```python
from build123d import *

# Parameters (mm, degrees)
F2_DEPTH = 12.7
F3_R     = 1.5875
F4_DEPTH = 12.701


# Not quite as in the source:
# - a feature names something its author has since deleted; it is built from what else it names


with BuildPart() as f2:
    # F1 (on face) → F2 (new body)
    with BuildSketch(Plane.YZ):
        Polygon((-152.4, -76.2), (139.7, -76.2), (139.7, 0), (152.4, 0), (152.4, 76.2), (-152.4, 76.2), (-207.8690637022, 76.2), align=None)
    extrude(amount=F2_DEPTH)

    # F3 (on face) → F4 (cut, through all)
    with BuildSketch(Plane.YZ):
        with Locations((-141.2875, 0)):
            Circle(F3_R)
        with Locations((88.9, 0)):
            Circle(F3_R)
    extrude(amount=F4_DEPTH, mode=Mode.SUBTRACT)


solid = f2.part
```
Could you check a few things on this model? Use its own coordinates, in mm. A direction names the side the tool comes from. Coordinates: 2 decimals unless noted, no trailing zeros. Write each loop counter-clockwise with the first axis right and the second up, starting at its lowest first coordinate (ties: lowest second). Pieces come first, ordered by that corner, then holes. Notation, with made-up numbers: (68, 49) - (110, 49) arc R23 ccw to (110, 67) - close; hole circle Ø10 at (75, 77). An arc over 180 degrees is marked (long way). Use a Markdown table: item, result.
Q1. Imagine slicing it at B-B (z = 41). List the corners of the cut face in (x, y) for me, and give its area (3 significant figures).
Geometry check:
| item | result |
|---|---|
| outline | (0, -195.06) - (12.7, -195.06) - (12.7, 152.4) - (0, 152.4) - close |
| area | 4,410 mm2 |
Q2. Which directions (+Z, -Z, +X, -X, +Y, -Y) give clear straight access to the entire face, cutting with the end or side of a thin tool? Please do faces 1 (the flat face through (0, -30, 1)), 2 (the flat face through (6, 139.7, -39)).
Geometry check:
| item | result |
|---|---|
| face 1 | +Z, -Z, -X, +Y, -Y |
| face 2 | -Z, +X, -X, +Y |
Q3. I'm going to push flat-ended pins straight in: pin 1 Ø3.5 at (y, z) = (88.9, 0) entering from -X; pin 2 Ø3 at (x, z) = (7.5, -4) entering from -Y; pin 3 Ø4 at (x, z) = (4.5, -47.5) entering from +Y; pin 4 Ø3 at (x, z) = (2.5, -57.5) entering from -Y. Where does each tip first touch, or does it pass through?
Geometry check:
| item | result |
|---|---|
| pin 1 | stops at x = 0 |
| pin 2 | stops at y = -179.22 |
| pin 3 | stops at y = 139.7 |
| pin 4 | stops at y = -159.75 |
Q4. Please list where these lines run through material, in increasing order: L1, parallel to Z at x = 10, y = 88.9; L2, parallel to Y at x = 7.25, z = 18; L3, parallel to Y at x = 7.5, z = 44.
Geometry check:
| item | result |
|---|---|
| L1 | z = -76.2 to -1.59, 1.59 to 76.2 |
| L2 | y = -186.69 to 152.4 |
| L3 | y = -196.15 to 152.4 |
Q5. Imagine slicing it at C-C (z = 59.5). List the corners of the cut face in (x, y) for me, and give its area (3 significant figures).
Geometry check:
| item | result |
|---|---|
| outline | (0, -201.79) - (12.7, -201.79) - (12.7, 152.4) - (0, 152.4) - close |
| area | 4,500 mm2 |
Q6. Imagine slicing it at A-A (x = 4). List the corners of the cut face in (y, z) for me (1 decimal).
Geometry check:
| item | result |
|---|---|
| outline | (-207.9, 76.2) - (-152.4, -76.2) - (139.7, -76.2) - (139.7, 0) - (152.4, 0) - (152.4, 76.2) - close; hole circle Ø3.2 at (-141.3, 0); hole circle Ø3.2 at (88.9, 0) |
